from build123d import *

# Parameters (mm, degrees)
SKETCH1_R           = 64
SKETCH1_R_2         = 55
SKETCH1_R_3         = 2.05
BOSS_EXTRUDE1_DEPTH = 6


with BuildPart() as part:
    # Sketch1 → Boss-Extrude1 (new body)
    with BuildSketch(Plane.XY):
        with Locations((-89.072792821, 47.25870832)):
            Circle(SKETCH1_R)
        with Locations((-89.072792821, 47.25870832)):
            Circle(SKETCH1_R_2, mode=Mode.SUBTRACT)
        with Locations((-32.08316907, 62.529031982)):
            Circle(SKETCH1_R_3, mode=Mode.SUBTRACT)
        with Locations((-32.08316907, 31.988384659)):
            Circle(SKETCH1_R_3, mode=Mode.SUBTRACT)
        with Locations((-47.353492731, 5.53940823)):
            Circle(SKETCH1_R_3, mode=Mode.SUBTRACT)
        with Locations((-73.80246916, -9.730915431)):
            Circle(SKETCH1_R_3, mode=Mode.SUBTRACT)
        with Locations((-104.343116482, -9.730915431)):
            Circle(SKETCH1_R_3, mode=Mode.SUBTRACT)
        with Locations((-130.792092911, 5.53940823)):
            Circle(SKETCH1_R_3, mode=Mode.SUBTRACT)
        with Locations((-146.062416572, 31.988384659)):
            Circle(SKETCH1_R_3, mode=Mode.SUBTRACT)
        with Locations((-146.062416572, 62.529031982)):
            Circle(SKETCH1_R_3, mode=Mode.SUBTRACT)
        with Locations((-130.792092911, 88.978008411)):
            Circle(SKETCH1_R_3, mode=Mode.SUBTRACT)
        with Locations((-104.343116482, 104.248332072)):
            Circle(SKETCH1_R_3, mode=Mode.SUBTRACT)
        with Locations((-73.80246916, 104.248332072)):
            Circle(SKETCH1_R_3, mode=Mode.SUBTRACT)
        with Locations((-47.353492731, 88.978008411)):
            Circle(SKETCH1_R_3, mode=Mode.SUBTRACT)
    extrude(amount=BOSS_EXTRUDE1_DEPTH)


solid = part.part
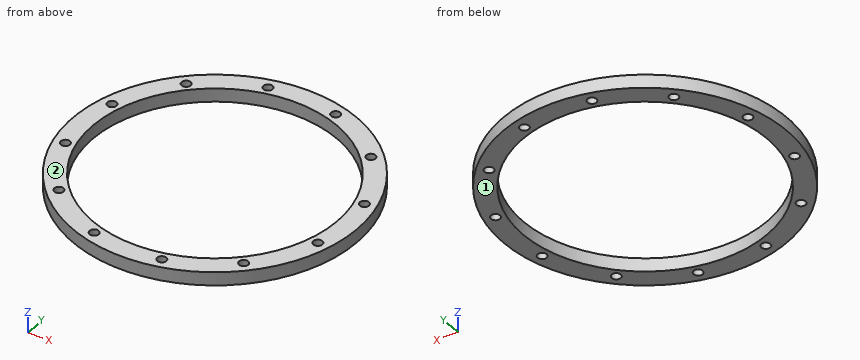
Design review of the part built by this model. Coordinates are the model's own, in mm. Face numbers are marked on the shaded views. Round coordinates to 2 decimals unless told otherwise and drop trailing zeros. Write each loop counter-clockwise with the first axis right and the second up, starting at its lowest first coordinate (ties: lowest second). Pieces come first, ordered by that corner, then holes.
Item 1: Draft analysis for pull direction Z (two halves, no side actions). For the marked faces 1 and 2, state which applies: released by +Z, released by -Z, zero draft, split by the parting line, or undercut.
Item 2: Wall thickness on L1, parallel to Y at x = -48.5, z = 3; L2, parallel to Y at x = -146.5, z = 5.2; L3, parallel to Y at x = -105, z = 0.9: over which ranges is each line inside the solid? List them lowest first.
Item 3: For pin 1 Ø1 at (x, z) = (-127.5, 0.5) entering from +Y, flat-tipped, find the tip position at first contact; note if it passes through.
Item 4: Consider section A-A on x = -86.5. Give the boundary of the cut face in (y, z).
Item 5: Consider section C-C on z = 2.7. Count the separate pieces of the cut face and the enclosed holes in it, and give its area (3 significant figures).
Item 6: Consider section B-B on y = 24.5. Give the boundary of the cut face in (x, z), and give its area (3 significant figures).
Check values:
1. face 1: released by -Z
1. face 2: released by +Z
2. L1: y = -2.24 to 3.84, 7.24 to 10.13, 84.39 to 87.28, 90.68 to 96.75
2. L2: y = 19.01 to 29.99, 33.99 to 60.53, 64.53 to 75.51
2. L3: y = -14.73 to -11.67, -7.79 to -5.38, 99.9 to 102.31, 106.19 to 109.25
3. pin 1: stops at y = 98.81
4. outline: (-16.69, 0) - (-7.68, 0) - (-7.68, 6) - (-16.69, 6) - close; (102.2, 0) - (111.21, 0) - (111.21, 6) - (102.2, 6) - close
5. separate pieces: 1
5. enclosed holes: 13
5. area: 3,210 mm2
6. outline: (-148.89, 0) - (-139.14, 0) - (-139.14, 6) - (-148.89, 6) - close; (-39, 0) - (-29.26, 0) - (-29.26, 6) - (-39, 6) - close
6. area: 117 mm2
